Input: part model. Units: mm. Frame: model coordinates. A direction names the side the tool comes from. Give positions to 0.01 mm unless a question says otherwise; leave off trailing zeros. Order: outer loops, then holes, each group sorted by start corner. A loop starts at its lowest first (then second) coordinate and runs counter-clockwise, first axis right, second up. Notation, with made-up numbers: (-13.75, -9) - (2.25, -9) arc R21 ccw to (2.25, 16) - close; hole circle Ø11 at (60.5, -37). An arc over 180 degrees is marked (long way). Use a Markdown table: item, result.
from build123d import *

# Parameters (mm, degrees)
F0_W     = 23.6095096916
F0_H     = 11.28009893
F1_DEPTH = 25.4
F2_W     = 67.4182642251
F2_H     = 11.28009893
F3_DEPTH = 12.7
F4_R     = 3.5729490202
F5_DEPTH = 25.4
F6_R     = 3.5729545
F7_DEPTH = 25.4


with BuildPart() as f1:
    # F0 (on Top) → F1 (new body)
    with BuildSketch(Plane.XY):
        with Locations((11.8047548458, -5.640049465)):
            Rectangle(F0_W, F0_H)
    extrude(amount=F1_DEPTH)

    # F2 (on face) → F3 (join)
    with BuildSketch(Plane.XY.offset(25.4)):
        with Locations((11.4112636074, -5.640049465)):
            Rectangle(F2_W, F2_H)
    extrude(amount=F3_DEPTH)

    # F4 (on face) → F5 (join)
    with BuildSketch(Plane.YZ.offset(45.12039572)):
        with Locations((-5.5088857189, 31.75)):
            Circle(F4_R)
    extrude(amount=F5_DEPTH)

    # F6 (on face) → F7 (join)
    with BuildSketch(Plane(origin=(-22.2978685051, 0, 0), x_dir=(0, -1, 0), z_dir=(-1, 0, 0))):
        with Locations((7.70714443, 31.75)):
            Circle(F6_R)
    extrude(amount=F7_DEPTH)


solid = f1.part
1. Set-up query: faces 1 (the face through (34, -6, 25.4)), 2 (the face through (57.64, -6.28, 28.26)), 3 (the face through (0, -6, 13)), 4 (the face through (-34.82, -6.933, 28.262)). Return all of +Z, -Z, +X, -X, +Y, -Y with unobstructed straight access to the full face (end or side cutting, diameter ignored); none if empty.
Response:
| item | result |
|---|---|
| face 1 | -Z, +X, +Y, -Y |
| face 2 | +X |
| face 3 | -Z, -X, +Y, -Y |
| face 4 | -X |
2. Material intervals for line 1 along Z through (x, y) = (-31, -7.5); line 2 along X through (y, z) = (-1, 3.5); line 3 along X through (y, z) = (-8, 26.5), sorted ascending.
Response:
| item | result |
|---|---|
| line 1 | z = 28.18 to 35.32 |
| line 2 | x = 0 to 23.61 |
| line 3 | x = -22.3 to 45.12 |
3. Section query A-A (x = -15.5). Return loops of the section in (y, z), then the cut area to 3 significant figures.
Response:
| item | result |
|---|---|
| outline | (-11.28, 25.4) - (0, 25.4) - (0, 38.1) - (-11.28, 38.1) - close |
| area | 143 mm^2 |
4. Pin query (flat end, axial travel): pin 1 (5.5 mm diameter, centred on x = -6, y = -4.5, fed in from -Z); pin 2 (4 mm diameter, centred on y = -2, z = 10, fed in from -X); pin 3 (5 mm diameter, centred on x = -34.5, y = -7, fed in from +Z); pin 4 (3 mm diameter, centred on x = -2, z = 33.5, fed in from +Y). Return the tip coordinate at first contact, or that it passes through.
Response:
| item | result |
|---|---|
| pin 1 | stops at z = 25.4 |
| pin 2 | stops at x = 0 |
| pin 3 | stops at z = 35.32 |
| pin 4 | stops at y = 0 |
5. Section query B-B (z = 9). Return loops of the section in (x, y), then the cut area to 3 significant figures.
Response:
| item | result |
|---|---|
| outline | (0, -11.28) - (23.61, -11.28) - (23.61, 0) - (0, 0) - close |
| area | 266 mm^2 |
6. Section query C-C (y = -3). Return loops of the section in (x, z), then the cut area to 3 significant figures.
Response:
| item | result |
|---|---|
| outline | (-22.3, 25.4) - (0, 25.4) - (0, 0) - (23.61, 0) - (23.61, 25.4) - (45.12, 25.4) - (45.12, 29.21) - (70.52, 29.21) - (70.52, 34.29) - (45.12, 34.29) - (45.12, 38.1) - (-22.3, 38.1) - close |
| area | 1,590 mm^2 |
